Verification items for the finished model (mm, model axes). Coordinates: 2 decimals unless noted, no trailing zeros. Answer as a JSON object with one key per item and string values. Group by question number.
Q1. Scan lines: L1, parallel to Y at x = -75, z = 1.5; L2, parallel to Y at x = -74, z = 0.3; L3, parallel to X at y = -41, z = 3.9. Record each from-to range of solid material in increasing order.
Q2. Gauge pin test, flat ends, axial feed: pin 1 Ø10 at (x, y) = (205, -120) entering from -Z; pin 2 Ø2.5 at (x, z) = (-209.5, 1.5) entering from -Y; pin 3 Ø1.5 at (x, z) = (196, 1.5) entering from +Y. Record the tip position at first contact, or that the pin passes through.
Q3. Cross-section at A-A on z = 0.85. Give the number of separate pieces and of enclosed holes in the cut face, and give its area (3 significant figures).
```python
from build123d import *

# Parameters (mm, degrees)
SKETCH_1_W          = 450
SKETCH_1_H          = 400
EXTRUDE_1_DEPTH     = 5
SKETCH_3_R          = 3.75
SKETCH_3_R_2        = 4.25
CUT_EXTRUDE_2_DEPTH = 50
SKETCH_5_W          = 45
SKETCH_5_H          = 45
CUT_EXTRUDE_4_DEPTH = 56
FILLET_1_R          = 5
SKETCH_6_R          = 4.25
CUT_EXTRUDE_5_DEPTH = 90
SKETCH_7_R          = 4.25
CUT_EXTRUDE_6_DEPTH = 90


with BuildPart() as part:
    # 草图1 → 凸台-拉伸1 (new body)
    with BuildSketch(Plane.XY):
        Rectangle(SKETCH_1_W, SKETCH_1_H)
    extrude(amount=EXTRUDE_1_DEPTH)

    # 草图3 → 切除-拉伸2 (cut)
    with BuildSketch(Plane.XY.offset(5)):
        with Locations((205, -180)):
            Circle(SKETCH_3_R)
        with Locations((205, -120)):
            Circle(SKETCH_3_R_2)
        with Locations((145, -180)):
            Circle(SKETCH_3_R_2)
        with Locations((145, 180)):
            Circle(SKETCH_3_R_2)
        with Locations((205, 120)):
            Circle(SKETCH_3_R_2)
        with Locations((205, 180)):
            Circle(SKETCH_3_R)
        with Locations((-205, 180)):
            Circle(SKETCH_3_R)
        with Locations((-205, 120)):
            Circle(SKETCH_3_R_2)
        with Locations((-145, 180)):
            Circle(SKETCH_3_R_2)
        with Locations((-145, -180)):
            Circle(SKETCH_3_R_2)
        with Locations((-205, -120)):
            Circle(SKETCH_3_R_2)
        with Locations((-205, -180)):
            Circle(SKETCH_3_R)
    extrude(amount=-CUT_EXTRUDE_2_DEPTH, mode=Mode.SUBTRACT)

    # 草图5 → 切除-拉伸4 (cut)
    with BuildSketch(Plane.XY.offset(5)):
        with Locations((202.5, -177.5)):
            Rectangle(SKETCH_5_W, SKETCH_5_H)
        with Locations((-202.5, -177.5)):
            Rectangle(SKETCH_5_W, SKETCH_5_H)
        with Locations((-202.5, 177.5)):
            Rectangle(SKETCH_5_W, SKETCH_5_H)
        with Locations((202.5, 177.5)):
            Rectangle(SKETCH_5_W, SKETCH_5_H)
    extrude(amount=-CUT_EXTRUDE_4_DEPTH, mode=Mode.SUBTRACT)

    # 圆角1
    fillet_1_edges = [part.edges().sort_by_distance(p)[0] for p in [
        (-180, -200, 2.5),
        (-225, -155, 2.5),
        (-180, -155, 2.5),
        (225, -155, 2.5),
        (180, -200, 2.5),
        (180, -155, 2.5),
        (180, 200, 2.5),
        (225, 155, 2.5),
        (180, 155, 2.5),
        (-225, 155, 2.5),
        (-180, 200, 2.5),
        (-180, 155, 2.5),
    ]]
    fillet(fillet_1_edges, radius=FILLET_1_R)

    # 草图6 → 切除-拉伸5 (cut)
    with BuildSketch(Plane(origin=(0, 0, 0), x_dir=(-1, 0, 0), z_dir=(0, 0, -1))):
        with Locations((75, -180)):
            Circle(SKETCH_6_R)
        with Locations((-75, -180)):
            Circle(SKETCH_6_R)
        with Locations((-75, -20)):
            Circle(SKETCH_6_R)
        with Locations((75, -20)):
            Circle(SKETCH_6_R)
    extrude(amount=-CUT_EXTRUDE_5_DEPTH, mode=Mode.SUBTRACT)

    # 草图7 → 切除-拉伸6 (cut)
    with BuildSketch(Plane(origin=(0, 0, 0), x_dir=(-1, 0, 0), z_dir=(0, 0, -1))):
        with Locations((-15, 180)):
            Circle(SKETCH_7_R)
        with Locations((-45, 180)):
            Circle(SKETCH_7_R)
        with Locations((-75, 180)):
            Circle(SKETCH_7_R)
        with Locations((-105, 180)):
            Circle(SKETCH_7_R)
        with Locations((-205, 12.5)):
            Circle(SKETCH_7_R)
        with Locations((-205, 37.5)):
            Circle(SKETCH_7_R)
        with Locations((-205, 62.5)):
            Circle(SKETCH_7_R)
        with Locations((-205, 87.5)):
            Circle(SKETCH_7_R)
        with Locations((-205, -87.5)):
            Circle(SKETCH_7_R)
        with Locations((-205, -62.5)):
            Circle(SKETCH_7_R)
        with Locations((-205, -37.5)):
            Circle(SKETCH_7_R)
        with Locations((-205, -12.5)):
            Circle(SKETCH_7_R)
        with Locations((205, -12.5)):
            Circle(SKETCH_7_R)
        with Locations((205, -37.5)):
            Circle(SKETCH_7_R)
        with Locations((205, -62.5)):
            Circle(SKETCH_7_R)
        with Locations((205, -87.5)):
            Circle(SKETCH_7_R)
        with Locations((205, 87.5)):
            Circle(SKETCH_7_R)
        with Locations((205, 62.5)):
            Circle(SKETCH_7_R)
        with Locations((205, 37.5)):
            Circle(SKETCH_7_R)
        with Locations((205, 12.5)):
            Circle(SKETCH_7_R)
        with Locations((105, 180)):
            Circle(SKETCH_7_R)
        with Locations((75, 180)):
            Circle(SKETCH_7_R)
        with Locations((45, 180)):
            Circle(SKETCH_7_R)
        with Locations((15, 180)):
            Circle(SKETCH_7_R)
        with Locations((15, -180)):
            Circle(SKETCH_7_R)
        with Locations((45, -180)):
            Circle(SKETCH_7_R)
        with Locations((75, -180)):
            Circle(SKETCH_7_R)
        with Locations((105, -180)):
            Circle(SKETCH_7_R)
        with Locations((-105, -180)):
            Circle(SKETCH_7_R)
        with Locations((-75, -180)):
            Circle(SKETCH_7_R)
        with Locations((-45, -180)):
            Circle(SKETCH_7_R)
        with Locations((-15, -180)):
            Circle(SKETCH_7_R)
    extrude(amount=-CUT_EXTRUDE_6_DEPTH, mode=Mode.SUBTRACT)


solid = part.part
```
Computed values:
{
 "1": {"L1": "y = -200 to -184.25, -175.75 to -24.25, -15.75 to 175.75, 184.25 to 200", "L2": "y = -200 to -184.13, -175.87 to -24.13, -15.87 to 175.87, 184.13 to 200", "L3": "x = -225 to -207.41, -202.59 to 202.59, 207.41 to 225"},
 "2": {"pin 1": "stops at z = 0", "pin 2": "stops at y = -155", "pin 3": "stops at y = 155"},
 "3": {"separate pieces": "1", "enclosed holes": "42", "area": "169,000 mm²"}
}
